```python
from build123d import *

# Parameters (mm, degrees)
SKETCH1_W                = 101.6
SKETCH1_H                = 25.4
BOSS_EXTRUDE1_DEPTH      = 2.54
BOSS_EXTRUDE2_DEPTH      = 19.05
BOSS_EXTRUDE2_DEPTH_BACK = 2.54
CUT_EXTRUDE1_DEPTH       = 3.81
CUT_EXTRUDE2_DEPTH       = 2.794
SKETCH5_W                = 101.6
SKETCH5_H                = 5.138615385
SKETCH5_H_2              = 5.275384615
CUT_EXTRUDE3_DEPTH       = 3.556
SKETCH6_R                = 1.651
CUT_EXTRUDE4_DEPTH       = 71.061780504


with BuildPart() as part:
    # Sketch1 → Boss-Extrude1 (new body)
    with BuildSketch(Plane(origin=(0, 0, 0), x_dir=(1, 0, 0), z_dir=(0, 1, 0))):
        with Locations((17.263096397, -7.815384615)):
            Rectangle(SKETCH1_W, SKETCH1_H)
    extrude(amount=BOSS_EXTRUDE1_DEPTH)

    # Sketch2 → Boss-Extrude2 (add, two sides: drawn at the far end of the back side and taken through both)
    with BuildSketch(Plane.XY.offset(-BOSS_EXTRUDE2_DEPTH_BACK)):
        Polygon((17.263096397, 2.54), (17.263096397, 5.588), (66.475596397, 5.588), (66.475596397, 2.54), (68.063096397, 2.54), (68.063096397, 7.1755), (-33.536903603, 7.1755), (-33.536903603, 2.54), align=None)
    extrude(amount=BOSS_EXTRUDE2_DEPTH + BOSS_EXTRUDE2_DEPTH_BACK)

    # Sketch3 → Cut-Extrude1 (cut)
    with BuildSketch(Plane.XY.offset(19.05)):
        Polygon((-33.536903603, 7.1755), (-33.536903603, 2.54), (17.263096397, 2.54), (17.263096397, 5.588), (66.475596397, 5.588), (66.475596397, 2.54), (68.063096397, 2.54), (68.063096397, 7.1755), align=None)
    extrude(amount=-CUT_EXTRUDE1_DEPTH, mode=Mode.SUBTRACT)

    # Sketch4 → Cut-Extrude2 (cut)
    with BuildSketch(Plane(origin=(0, 0, -2.54), x_dir=(-1, 0, 0), z_dir=(0, 0, -1))):
        Polygon((-68.063096397, 7.1755), (-68.063096397, 2.54), (-66.475596397, 2.54), (-66.475596397, 5.588), (-17.263096397, 5.588), (-17.263096397, 2.54), (33.536903603, 2.54), (33.536903603, 7.1755), align=None)
    extrude(amount=-CUT_EXTRUDE2_DEPTH, mode=Mode.SUBTRACT)

    # Sketch5 → Cut-Extrude3 (cut)
    with BuildSketch(Plane(origin=(0, 2.54, 0), x_dir=(1, 0, 0), z_dir=(0, 1, 0))):
        with Locations((17.263096397, 2.315307693)):
            Rectangle(SKETCH5_W, SKETCH5_H)
        with Locations((17.263096397, -17.877692308)):
            Rectangle(SKETCH5_W, SKETCH5_H_2)
    extrude(amount=-CUT_EXTRUDE3_DEPTH, mode=Mode.SUBTRACT)

    # Sketch6 → Cut-Extrude4 (cut, through all)
    with BuildSketch(Plane.XY.offset(15.24)):
        with Locations((-29.726903603, 4.064)):
            Circle(SKETCH6_R)
    extrude(amount=-CUT_EXTRUDE4_DEPTH, mode=Mode.SUBTRACT)


solid = part.part
```
The listing builds one solid part. Answer for the finished solid, in the listing's coordinates (mm). A direction names the side the tool comes from. Give positions to 0.01 mm unless a question says otherwise; leave off trailing zeros. Loops run counter-clockwise (first coordinate to the right, second up) from the corner with the lowest first, then second, coordinate; pieces in that order, holes last. Notation, with made-up numbers: M 86,-20.5 L 126,-20.5 A20 ccw 126,0.5 Z; hole C 32,82.5 d11. An arc over 180 degrees is marked long. One line per item, written item: value.
Q1. Find the intervals of material crossed by line 1 (X direction, y = 4, z = 12.5); line 2 (Y direction, x = 22, z = 8.75); line 3 (X direction, y = 3.5, z = 10.5), in increasing order. Write a range as from..to.
Working result:
line 1: x = -33.54..-31.38, -28.08..17.26, 66.48..68.06
line 2: y = 0..2.54, 5.59..7.18
line 3: x = -33.54..-31.28, -28.18..17.26, 66.48..68.06
Q2. A cutting plane is placed at B-B on z = 4.25. Determine the outline of the cut face in (x, y).
Working result:
outline: M -33.54,0 L 68.06,0 L 68.06,7.18 L -33.54,7.18 Z; hole C -29.73,4.06 d3.3; hole M 17.26,2.54 L 66.48,2.54 L 66.48,5.59 L 17.26,5.59 Z
Q3. A cutting plane is placed at A-A on x = 31. Determine the outline of the cut face in (y, z).
Working result:
outline: M 0,0.25 L 2.54,0.25 L 2.54,15.24 L 0,15.24 Z; M 5.59,0.25 L 7.18,0.25 L 7.18,15.24 L 5.59,15.24 Z
Q4. Determine the mould class of faces 1 (the face through (17, 0, 8)), 2 (the face through (-33.537, 4, 8)), 3 (the face through (42, 2.54, 8)) for opening direction X: +X half, -X half, draft (parallel to the pull), parting line (faces both ways), or undercut.
Working result:
face 1: draft
face 2: -X half
face 3: undercut
Q5. For faces 4 (the face through (17.263, 4, 8)), 5 (the face through (18, 7.176, 8)), determine the directions among +Z, -Z, +X, -X, +Y, -Y from which every point of the face is accessible in a straight line to the end or side of a thin tool.
Working result:
face 4: +Z, -Z
face 5: +Z, -Z, +X, -X, +Y
